Autodesk Inventor part; units mm, degrees
ref_plane "YZ Plane" through (0, 0, 0) normal (1, 0, 0) x (0, 1, 0)
ref_plane "XZ Plane" through (0, 0, 0) normal (0, 1, 0) x (-1, 0, 0)
ref_plane "XY Plane" through (0, 0, 0) normal (0, 0, 1) x (1, 0, 0)
sketch "Эскиз1" plane through (0, 0, 0) normal (0, 1, 0) x (-1, 0, 0)
  line L0 (21.1, -21.1) -> (-21.1, -21.1)
  line L1 (-21.1, -21.1) -> (-21.1, 21.1)
  line L2 (-21.1, 21.1) -> (21.1, 21.1)
  line L3 (21.1, 21.1) -> (21.1, -21.1)
  line L4 (21.1, -21.1) -> (-21.1, 21.1) construction
  line L5 (-21.1, -21.1) -> (21.1, 21.1) construction
  line L6 (-15.55, 15.55) -> (15.55, 15.55) construction
  line L7 (15.55, 15.55) -> (15.55, -15.55) construction
  line L8 (15.55, -15.55) -> (-15.55, -15.55) construction
  line L9 (-15.55, -15.55) -> (-15.55, 15.55) construction
  line L10 (-15.55, 15.55) -> (15.55, -15.55) construction
  line L11 (15.55, 15.55) -> (-15.55, -15.55) construction
  circle A0 centre (-15.55, -15.55) radius 1.5
  circle A1 centre (15.55, -15.55) radius 1.5
  circle A2 centre (15.55, 15.55) radius 1.5
  circle A3 centre (-15.55, 15.55) radius 1.5
  point P0 (0, 0)
  dimension "d0" = 42.2
  dimension "d1" = 42.2
  dimension "d2" = 31.1
  dimension "d3" = 31.1
  dimension "d4" = 3
  dimension "d5" = 3
  dimension "d6" = 3
  dimension "d7" = 3
extrude "Выдавливание1" add sketch "Эскиз1" along normal blind 8
sketch "Эскиз2" plane through (0, 8, 0) normal (0, 1, 0) x (1, 0, 0)
  circle A0 centre (0, 0) radius 11
  dimension "d10" = 22
extrude "Выдавливание2" add sketch "Эскиз2" along normal blind 2
chamfer "Фаска1" distance 4.5 angle 45 4 edges at (21.1, 4, -21.1) (21.1, 4, 21.1) (-21.1, 4, 21.1) (-21.1, 4, -21.1)
sketch "Эскиз3" plane through (0, 10, 0) normal (0, 1, 0) x (1, 0, 0)
  circle A0 centre (0, 0) radius 11
  circle A1 centre (0, 0) radius 5
  dimension "d16" = 10
extrude "Выдавливание3" cut sketch "Эскиз3" against normal blind 9 contours A1
thread "Резьба1"
thread "Резьба2"
thread "Резьба3"
thread "Резьба4"
properties part number "Top"
Work out the finished part from the listing and answer in its coordinate system (mm). A direction names the side the tool comes from. Coordinates: 2 decimals unless noted, no trailing zeros. Write each loop counter-clockwise with the first axis right and the second up, starting at its lowest first coordinate (ties: lowest second). Pieces come first, ordered by that corner, then holes. Notation, with made-up numbers: M 24.5,-17.5 L 28.5,-17.5 A22 ccw 28.5,5.5 Z; hole C 45.25,56.25 d6. An arc over 180 degrees is marked long. Use one line per item in the form item = value. Start each with the question number.
1. The part is cut by section D-D (x = 0). Give the vertices of the cut face in (y, z), plus the area to 3 significant figures.
2. The part is cut by section C-C (x = 15.55). Give the vertices of the cut face in (y, z), plus the area to 3 significant figures.
3. The part is cut by section A-A (y = 2.75). Give the vertices of the cut face in (x, z), plus the area to 3 significant figures.
4. The part is cut by section B-B (z = -15.55). Give the vertices of the cut face in (x, y), plus the area to 3 significant figures.
5. Each of these flat-tipped pins is pushed along its axis until it touches: P1, Ø3.5, axis at x = 15.55, z = -15.55, coming from the +Y side; P2, Ø1.8, axis at x = -15.55, z = -15.55, coming from the -Y side. Where does it stop, or does it pass through?
6. Straight lines are drawn through the part: probe 1 along Z at (x, y) = (15.5, 0.5); probe 2 along X at (y, z) = (5, 0); probe 3 along Y at (x, z) = (0, -18). For each, find the intervals that lie inside material, in ascending order. Write a range as from..to.
7. The mould has two halves that part along X. Classify faces 1 (the face through (0, 1, 0)), 2 (the face through (0, 0, 0)), 3 (the face through (-2.38, 8.99, -10.74)): released by +X, released by -X, zero draft, split by the parting line, or undercut.
8. A tool of negligible diameter and unlimited length cuts with its end or side. For faces 4 (the face through (-9, 8, -9)), 5 (the face through (15.875, 3.944, -14.086)), from which of +Z, -Z, +X, -X, +Y, -Y can it reach the whole face along a straight path? Write none if from no direction.
Evaluation:
q1.outline = M 0,-21.1 L 8,-21.1 L 8,-11 L 10,-11 L 10,-5 L 1,-5 L 1,5 L 10,5 L 10,11 L 8,11 L 8,21.1 L 0,21.1 Z
q1.area = 292 mm^2
q2.outline = M 0,-21.1 L 8,-21.1 L 8,-17.05 L 0,-17.05 Z; M 0,-14.05 L 8,-14.05 L 8,14.05 L 0,14.05 Z; M 0,17.05 L 8,17.05 L 8,21.1 L 0,21.1 Z
q2.area = 290 mm^2
q3.outline = M -21.1,-16.6 L -16.6,-21.1 L 16.6,-21.1 L 21.1,-16.6 L 21.1,16.6 L 16.6,21.1 L -16.6,21.1 L -21.1,16.6 Z; hole C -15.55,-15.55 d3; hole C -15.55,15.55 d3; hole C 0,0 d10; hole C 15.55,-15.55 d3; hole C 15.55,15.55 d3
q3.area = 1,630 mm^2
q4.outline = M -21.1,0 L -17.05,0 L -17.05,8 L -21.1,8 Z; M -14.05,0 L 14.05,0 L 14.05,8 L -14.05,8 Z; M 17.05,0 L 21.1,0 L 21.1,8 L 17.05,8 Z
q4.area = 290 mm^2
q5.P1 = 8
q5.P2 = through
q6.probe_1 = -21.1..-17.05, -14.05..14.05, 17.05..21.1
q6.probe_2 = -21.1..-5, 5..21.1
q6.probe_3 = 0..8
q7.face_1 = undercut
q7.face_2 = zero draft
q7.face_3 = split by the parting line
q8.face_4 = +Y
q8.face_5 = +Y, -Y
